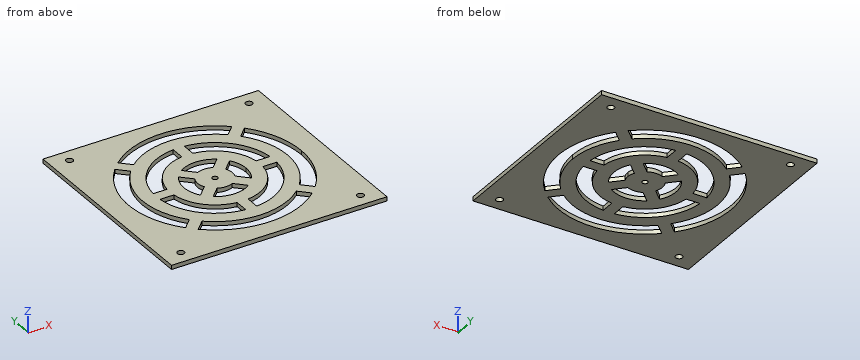
from build123d import *

# Parameters (mm, degrees)
SKETCH1_W           = 150
SKETCH1_H           = 150
BOSS_EXTRUDE1_DEPTH = 3
CUT_EXTRUDE1_DEPTH  = 264.0332057
SKETCH4_R           = 2.5
CUT_EXTRUDE2_DEPTH  = 3
SKETCH5_W           = 3
SKETCH5_H           = 150
BOSS_EXTRUDE2_DEPTH = 3
SKETCH6_R           = 2
CUT_EXTRUDE3_DEPTH  = 10


with BuildPart() as part:
    # Sketch1 → Boss-Extrude1 (new body)
    with BuildSketch(Plane.XY):
        with Locations((146.896551724, 66.206896552)):
            Rectangle(SKETCH1_W, SKETCH1_H)
    extrude(amount=BOSS_EXTRUDE1_DEPTH)

    # Sketch2 → Cut-Extrude1 (cut, through all)
    with BuildSketch(Plane.XY.offset(3)):
        with BuildLine():
            ThreePointArc((188.163122783, 113.13032186), (146.896551724, 128.694797217), (105.629980666, 113.13032186))
            Line((105.629980666, 113.13032186), (112.718359737, 106.041942789))
            ThreePointArc((112.718359737, 106.041942789), (146.896551724, 118.694797217), (181.074743712, 106.041942789))
            Line((181.074743712, 106.041942789), (188.163122783, 113.13032186))
        make_face()
        with BuildLine():
            Line((107.061505487, 100.385088539), (99.973126416, 107.47346761))
            ThreePointArc((99.973126416, 107.47346761), (84.408651059, 66.206896552), (99.973126416, 24.940325493))
            Line((99.973126416, 24.940325493), (107.061505487, 32.028704564))
            ThreePointArc((107.061505487, 32.028704564), (94.408651059, 66.206896552), (107.061505487, 100.385088539))
        make_face()
        with BuildLine():
            ThreePointArc((209.384452389, 66.206896552), (205.363995952, 88.259009716), (193.819977032, 107.47346761))
            Line((193.819977032, 107.47346761), (186.731597961, 100.385088539))
            ThreePointArc((186.731597961, 100.385088539), (196.119705149, 84.429434333), (199.384452389, 66.206896552))
            ThreePointArc((199.384452389, 66.206896552), (196.119705149, 47.984358771), (186.731597961, 32.028704564))
            Line((186.731597961, 32.028704564), (193.819977032, 24.940325493))
            ThreePointArc((193.819977032, 24.940325493), (205.363995952, 44.154783387), (209.384452389, 66.206896552))
        make_face()
        with BuildLine():
            Line((112.718359737, 26.371850315), (105.629980666, 19.283471244))
            ThreePointArc((105.629980666, 19.283471244), (146.896551724, 3.718995886), (188.163122783, 19.283471244))
            Line((188.163122783, 19.283471244), (181.074743712, 26.371850315))
            ThreePointArc((181.074743712, 26.371850315), (146.896551724, 13.718995886), (112.718359737, 26.371850315))
        make_face()
        with BuildLine():
            ThreePointArc((150.896551724, 23.907703853), (176.940034403, 36.163413873), (189.195744423, 62.206896552))
            Line((189.195744423, 62.206896552), (179.137266506, 62.206896552))
            ThreePointArc((179.137266506, 62.206896552), (169.868966591, 43.234481685), (150.896551724, 33.96618177))
            Line((150.896551724, 33.96618177), (150.896551724, 23.907703853))
        make_face()
        with BuildLine():
            Line((114.655836942, 62.206896552), (104.597359026, 62.206896552))
            ThreePointArc((104.597359026, 62.206896552), (116.853069045, 36.163413873), (142.896551724, 23.907703853))
            Line((142.896551724, 23.907703853), (142.896551724, 33.96618177))
            ThreePointArc((142.896551724, 33.96618177), (123.924136857, 43.234481685), (114.655836942, 62.206896552))
        make_face()
        with BuildLine():
            Line((142.896551724, 98.447611333), (142.896551724, 108.50608925))
            ThreePointArc((142.896551724, 108.50608925), (116.853069045, 96.250379231), (104.597359026, 70.206896552))
            Line((104.597359026, 70.206896552), (114.655836942, 70.206896552))
            ThreePointArc((114.655836942, 70.206896552), (123.924136857, 89.179311419), (142.896551724, 98.447611333))
        make_face()
        with BuildLine():
            ThreePointArc((189.195744423, 70.206896552), (176.940034403, 96.250379231), (150.896551724, 108.50608925))
            Line((150.896551724, 108.50608925), (150.896551724, 98.447611333))
            ThreePointArc((150.896551724, 98.447611333), (169.868966591, 89.179311419), (179.137266506, 70.206896552))
            Line((179.137266506, 70.206896552), (189.195744423, 70.206896552))
        make_face()
        with BuildLine():
            Line((165.372753073, 79.026243651), (158.090015102, 71.74350568))
            ThreePointArc((158.090015102, 71.74350568), (159.056537781, 69.049853135), (159.384452389, 66.206896552))
            ThreePointArc((159.384452389, 66.206896552), (159.166880972, 63.885973637), (158.521748029, 61.645923641))
            Line((158.521748029, 61.645923641), (165.932760465, 54.234911206))
            ThreePointArc((165.932760465, 54.234911206), (168.504305512, 59.977076926), (169.384452389, 66.206896552))
            ThreePointArc((169.384452389, 66.206896552), (168.358106385, 72.923096956), (165.372753073, 79.026243651))
        make_face()
        with BuildLine():
            Line((134.077204625, 84.6830979), (141.359942596, 77.400359929))
            ThreePointArc((141.359942596, 77.400359929), (146.896551724, 78.694797217), (152.433160852, 77.400359929))
            Line((152.433160852, 77.400359929), (159.715898823, 84.6830979))
            ThreePointArc((159.715898823, 84.6830979), (146.896551724, 88.694797217), (134.077204625, 84.6830979))
        make_face()
        with BuildLine():
            ThreePointArc((135.703088346, 60.670287424), (134.408651059, 66.206896552), (135.703088346, 71.74350568))
            Line((135.703088346, 71.74350568), (128.420350375, 79.026243651))
            ThreePointArc((128.420350375, 79.026243651), (124.408651059, 66.206896552), (128.420350375, 53.387549452))
            Line((128.420350375, 53.387549452), (135.703088346, 60.670287424))
        make_face()
        with BuildLine():
            ThreePointArc((152.433160852, 55.013433174), (146.896551724, 53.718995886), (141.359942596, 55.013433174))
            Line((141.359942596, 55.013433174), (134.077204625, 47.730695203))
            ThreePointArc((134.077204625, 47.730695203), (146.896551724, 43.718995886), (159.715898823, 47.730695203))
            Line((159.715898823, 47.730695203), (152.433160852, 55.013433174))
        make_face()
    extrude(amount=-CUT_EXTRUDE1_DEPTH, mode=Mode.SUBTRACT)

    # Sketch4 → Cut-Extrude2 (cut)
    with BuildSketch(Plane.XY.offset(3)):
        with Locations((81.896551724, 131.206896552)):
            Circle(SKETCH4_R)
        with Locations((211.896551724, 131.206896552)):
            Circle(SKETCH4_R)
        with Locations((211.896551724, 1.206896552)):
            Circle(SKETCH4_R)
        with Locations((81.896551724, 1.206896552)):
            Circle(SKETCH4_R)
    extrude(amount=-CUT_EXTRUDE2_DEPTH, mode=Mode.SUBTRACT)

    # Sketch5 → Boss-Extrude2 (add)
    with BuildSketch(Plane(origin=(0, 0, 0), x_dir=(-1, 0, 0), z_dir=(0, 0, -1))):
        with Locations((-223.396551724, 66.206896552)):
            Rectangle(SKETCH5_W, SKETCH5_H)
        with Locations((-70.396551724, 66.206896552)):
            Rectangle(SKETCH5_W, SKETCH5_H)
    extrude(amount=-BOSS_EXTRUDE2_DEPTH)

    # Sketch6 → Cut-Extrude3 (cut)
    with BuildSketch(Plane.XY.offset(3)):
        with Locations((146.896551724, 66.206896552)):
            Circle(SKETCH6_R)
    extrude(amount=-CUT_EXTRUDE3_DEPTH, mode=Mode.SUBTRACT)


solid = part.part
CAD build for the part. Positions are in the model's coordinates, mm. Give positions to 0.01 mm unless a question says otherwise; leave off trailing zeros. Order: outer loops, then holes, each group sorted by start corner. A loop starts at its lowest first (then second) coordinate and runs counter-clockwise, first axis right, second up. Notation, with made-up numbers: (79, -39.75) - (113, -39.75) arc R20 ccw to (113, -10.75) - close; hole circle Ø3 at (28.5, 32.25). An arc over 180 degrees is marked (long way). Write each question's results on one line, items separated by ' | '.
1. Saw through at A-A on x = 191.5. List the corners of the cut face in (y, z).
Calculated:
outline: (-8.79, 0) - (27.26, 0) - (27.26, 3) - (-8.79, 3) - close; (38.54, 0) - (93.87, 0) - (93.87, 3) - (38.54, 3) - close; (105.15, 0) - (141.21, 0) - (141.21, 3) - (105.15, 3) - close
2. Saw through at B-B on y = 81.5. List the corners of the cut face in (x, z), and give its area (3 significant figures).
Calculated:
outline: (68.9, 0) - (86.31, 0) - (86.31, 3) - (68.9, 3) - close; (96.69, 0) - (107.26, 0) - (107.26, 3) - (96.69, 3) - close; (118.23, 0) - (137.26, 0) - (137.26, 3) - (118.23, 3) - close; (156.53, 0) - (175.56, 0) - (175.56, 3) - (156.53, 3) - close; (186.54, 0) - (197.11, 0) - (197.11, 3) - (186.54, 3) - close; (207.48, 0) - (224.9, 0) - (224.9, 3) - (207.48, 3) - close | area: 282 mm2
3. Saw through at C-C on x = 117. List the corners of the cut face in (y, z), and give its area (3 significant figures).
Calculated:
outline: (-8.79, 0) - (11.33, 0) - (11.33, 3) - (-8.79, 3) - close; (23.07, 0) - (36.02, 0) - (36.02, 3) - (23.07, 3) - close; (53.49, 0) - (78.92, 0) - (78.92, 3) - (53.49, 3) - close; (96.4, 0) - (109.35, 0) - (109.35, 3) - (96.4, 3) - close; (121.08, 0) - (141.21, 0) - (141.21, 3) - (121.08, 3) - close | area: 275 mm2
4. Pin check, flat tip, straight feed: pin 1 (3 mm diameter, centred on x = 146.9, y = 66.21, fed in from +Z). Stop position of the tip, or through.
Calculated:
pin 1: passes through
5. Saw through at D-D on y = 126. List the corners of the cut face in (x, z), and give its area (3 significant figures).
Calculated:
outline: (68.9, 0) - (128.74, 0) - (128.74, 3) - (68.9, 3) - close; (165.05, 0) - (224.9, 0) - (224.9, 3) - (165.05, 3) - close | area: 359 mm2
6. Probe L1, parallel to X at y = 2, z = 1.6; L2, parallel to Y at x = 133, z = 2.15; L3, parallel to Y at x = 162.5, z = 1.6. List the from-to ranges inside material, lowest first. Write a range as from..to.
Calculated:
L1: x = 68.9..79.53, 84.27..209.53, 214.27..224.9 | L2: y = -8.79..5.28, 15.59..26.06, 36.84..57.97, 74.45..95.57, 106.36..116.82, 127.13..141.21 | L3: y = -8.79..5.7, 16.09..26.69, 37.71..57.67, 76.15..94.7, 105.73..116.32, 126.72..141.21
